```python
from build123d import *

# Parameters (mm, degrees)
F1_DEPTH = 7
F2_DEPTH = 7
F3_R     = 5


with BuildPart() as f1:
    # F0 (on Top) → F1 (new body)
    with BuildSketch(Plane.XY):
        Polygon((13.249245, 35.047099), (-13.2, 35.047099), (-13.2, 7.677887), (-36.976301, -6.049366), (-23.751678, -28.955085), (-0.049245, -15.270479), (23.727055, -28.997733), (36.951678, -6.092014), (13.249245, 7.592592), align=None)
        with BuildLine():
            ThreePointArc((-11.2, 0), (0, 11.2), (11.2, 0))
            ThreePointArc((11.2, 0), (0, -11.2), (-11.2, 0))
        make_face(mode=Mode.SUBTRACT)
    extrude(amount=F1_DEPTH)

    # F0 (on Top) → F2 (join)
    with BuildSketch(Plane.XY):
        Polygon((13.249245, 35.047099), (-13.2, 35.047099), (-13.2, 7.677887), (-36.976301, -6.049366), (-23.751678, -28.955085), (-0.049245, -15.270479), (23.727055, -28.997733), (36.951678, -6.092014), (13.249245, 7.592592), align=None)
        with BuildLine():
            ThreePointArc((-11.2, 0), (0, 11.2), (11.2, 0))
            ThreePointArc((11.2, 0), (0, -11.2), (-11.2, 0))
        make_face(mode=Mode.SUBTRACT)
    extrude(amount=F2_DEPTH)

    # F3
    f3_edges = [f1.edges().sort_by_distance(p)[0] for p in [
        (-13.2, 35.047099, 3.5),
        (13.249245, 35.047099, 3.5),
        (36.951678, -6.092014, 3.5),
        (23.727055, -28.997733, 3.5),
        (-23.751678, -28.955085, 3.5),
        (-36.976301, -6.049366, 3.5),
    ]]
    fillet(f3_edges, radius=F3_R)


solid = f1.part
```
Can you work these out from the model? Positions are in its coordinate system, mm. A direction names the side the tool comes from. Coordinates: 2 decimals unless noted, no trailing zeros. Order: outer loops, then holes, each group sorted by start corner. A loop starts at its lowest first (then second) coordinate and runs counter-clockwise, first axis right, second up.
1. For faces 4 (the face through (-13.2, 19, 3)), 5 (the face through (13.249, 19, 3)), 6 (the face through (9.538, -20.806, 3.451)), which set-ups out of +Z, -Z, +X, -X, +Y, -Y let a thin tool reach every point of the face, with its end or its side?
2. If we section it at C-C (x = -4): Please give me the cut outline in (y, z), then the cut area to 3 significant figures.
3. If we section it at D-D (y = 16.5): Please give me the cut outline in (x, z), then the cut area to 3 significant figures.
4. I'm going to push flat-ended pins straight in: pin 1 (1 mm diameter, centred on x = -17, z = 6, fed in from +Y); pin 2 (2 mm diameter, centred on y = 23.5, z = 2, fed in from -X); pin 3 (3.5 mm diameter, centred on y = 20, z = 2, fed in from +X). Where does each tip first touch, or does it pass through?
5. If we section it at A-A (z = 6): Please give me the cut outline in (x, y).
6. I need wall thicknesses on line 1 (X direction, y = 0, z = 5); line 2 (X direction, y = 13.5, z = 6.75); line 3 (Y direction, x = 0, z = 4). Which ranges of each line are inside material? Lowest first, please.
7. Thinking about a two-plate mould opening in X: for faces 1 (the face through (30.282, -17.645, 3.451)), 2 (the face through (-34.96, -6.53, 3.55)), 3 (the face through (-9.87, -20.94, 3.45)), which applies, +X half, -X half, draft (parallel to the pull), parting line (faces both ways), or undercut?
8. If we section it at B-B (y = -7): Please give me the cut outline in (x, z), then the cut area to 3 significant figures.
Entries:
1. face 4: +Z, -Z, -X, +Y
1. face 5: +Z, -Z, +X, +Y
1. face 6: +Z, -Z, -Y
2. outline: (-17.55, 0) - (-10.46, 0) - (-10.46, 7) - (-17.55, 7) - close; (10.46, 0) - (35.05, 0) - (35.05, 7) - (10.46, 7) - close
2. area: 222 mm2
3. outline: (-13.2, 0) - (13.25, 0) - (13.25, 7) - (-13.2, 7) - close
3. area: 185 mm2
4. pin 1: stops at y = 5.77
4. pin 2: stops at x = -13.2
4. pin 3: stops at x = 13.25
5. outline: (-34.48, -10.38) - (-26.25, -24.62) arc R5 ccw to (-19.42, -26.46) - (-0.05, -15.27) - (19.4, -26.5) arc R5 ccw to (26.23, -24.67) - (34.45, -10.42) arc R5 ccw to (32.62, -3.59) - (13.25, 7.59) - (13.25, 30.05) arc R5 ccw to (8.25, 35.05) - (-8.2, 35.05) arc R5 ccw to (-13.2, 30.05) - (-13.2, 7.68) - (-32.65, -3.55) arc R5 ccw to start; hole circle Ø22.4 at (0, 0)
6. line 1: x = -26.5 to -11.2, 11.2 to 26.4
6. line 2: x = -13.2 to 13.25
6. line 3: y = -15.3 to -11.2, 11.2 to 35.05
7. face 1: +X half
7. face 2: -X half
7. face 3: undercut
8. outline: (-35.07, 0) - (-8.74, 0) - (-8.74, 7) - (-35.07, 7) - close; (8.74, 0) - (35.04, 0) - (35.04, 7) - (8.74, 7) - close
8. area: 368 mm2
